Autodesk Inventor part; units mm, degrees
ref_plane "YZ Plane" through (0, 0, 0) normal (1, 0, 0) x (0, 1, 0)
ref_plane "XZ Plane" through (0, 0, 0) normal (0, 1, 0) x (-1, 0, 0)
ref_plane "XY Plane" through (0, 0, 0) normal (0, 0, 1) x (1, 0, 0)
sketch "Sketch1" plane through (0, 0, 0) normal (0, 1, 0) x (-1, 0, 0)
  point P0 (0, 0)
sketch "Sketch2" plane through (0, 0, 0) normal (0, 1, 0) x (-1, 0, 0)
  line L0 (38.1, 25.4) -> (-38.1, 25.4)
  line L1 (-38.1, 25.4) -> (-38.1, -25.4)
  line L2 (-38.1, -25.4) -> (38.1, -25.4)
  line L3 (38.1, -25.4) -> (38.1, 25.4)
  line L4 (34.798, 22.098) -> (-34.798, 22.098)
  line L5 (-34.798, 22.098) -> (-34.798, -22.098)
  line L6 (-34.798, -22.098) -> (34.798, -22.098)
  line L7 (34.798, -22.098) -> (34.798, 22.098)
  line L8 (0, -35.56) -> (0, 35.56)
  line L9 (-53.34, 0) -> (53.34, 0)
  point P0 (0, 0)
  dimension "d0" = 3.302
  dimension "d1" = 76.2
  dimension "d2" = 50.8
extrude "Extrusion1" add sketch "Sketch2" along normal mid plane 50.8 contours L3 L9 L7 L4 L8 L0 | L8 L4 L5 L9 L1 L0 | L3 L2 L8 L6 L7 L9 | L9 L5 L6 L8 L2 L1
sketch "Sketch3" plane through (-38.1, -25.4, 25.4) normal (0, 0, 1) x (1, 0, 0)
  circle A0 centre (25.4, 25.4) radius 14.2875
  line L0 (-15.24, 25.4) -> (91.44, 25.4)
  line L1 (38.1, 60.96) -> (38.1, -10.16)
  line L2 (0, 50.8) -> (0, 0)
  point P0 (38.1, 25.4)
  dimension "d5" = 28.575
  dimension "d6" = 25.4
extrude "Extrusion2" cut sketch "Sketch3" against normal up to surface (50.8 mm away)
properties part number "Hinge"
Could you check a few things on this model? Use its own coordinates, in mm. A direction names the side the tool comes from. Give positions to 0.01 mm unless a question says otherwise; leave off trailing zeros. Order: outer loops, then holes, each group sorted by start corner. A loop starts at its lowest first (then second) coordinate and runs counter-clockwise, first axis right, second up.
Q1. For faces 1 (the flat face through (8, 0, 25.4)), 2 (the flat face through (-34.798, 0, 0)), which set-ups out of +Z, -Z, +X, -X, +Y, -Y let a thin tool reach every point of the face, with its end or its side?
Q2. Suppose I cut it at A-A, the plane z = 4.5. Write out the boundary of the cut face in (x, y).
Q3. Suppose I cut it at B-B, the plane x = 8. Write out the boundary of the cut face in (y, z).
Q4. Suppose I cut it at C-C, the plane y = 0. Write out the boundary of the cut face in (x, z).
Q5. Suppose I cut it at D-D, the plane y = 20. Write out the boundary of the cut face in (x, z), and give its area (3 significant figures).
Q6. We'd pull the mould along Y, two halves only. Please class faces 3 (the cylindrical face through (0.93, 4.29, 23.77)), 4 (the cylindrical face through (0.93, 4.29, -23.73)), 5 (the flat face through (3, 25.4, -22.5)), 6 (the flat face through (38.1, 0, 0)): +Y half, -Y half, draft (parallel to the pull), parting line (faces both ways), or undercut.
Q7. If I drill on line 1 along Z through (x, y) = (27.5, 21); line 2 along X through (y, z) = (-11, -4.5); line 3 along X through (y, z) = (0, 23), over which ranges is the centre line in solid material (lowest first)?
Solution:
1. face 1: +Z, +X, -X, +Y, -Y
1. face 2: +Y, -Y
2. outline: (-38.1, -25.4) - (-34.8, -25.4) - (-34.8, 25.4) - (-38.1, 25.4) - close; (34.8, -25.4) - (38.1, -25.4) - (38.1, 25.4) - (34.8, 25.4) - close
3. outline: (-25.4, -25.4) - (25.4, -25.4) - (25.4, -22.1) - (-25.4, -22.1) - close; (-25.4, 22.1) - (25.4, 22.1) - (25.4, 25.4) - (-25.4, 25.4) - close
4. outline: (-38.1, -25.4) - (-26.99, -25.4) - (-26.99, -22.1) - (-34.8, -22.1) - (-34.8, 22.1) - (-26.99, 22.1) - (-26.99, 25.4) - (-38.1, 25.4) - close; (1.59, -25.4) - (38.1, -25.4) - (38.1, 25.4) - (1.59, 25.4) - (1.59, 22.1) - (34.8, 22.1) - (34.8, -22.1) - (1.59, -22.1) - close
5. outline: (-38.1, -25.4) - (38.1, -25.4) - (38.1, 25.4) - (-38.1, 25.4) - close; hole (-34.8, -22.1) - (34.8, -22.1) - (34.8, 22.1) - (-34.8, 22.1) - close
5. area: 795 mm2
6. face 3: undercut
6. face 4: undercut
6. face 5: +Y half
6. face 6: draft
7. line 1: z = -25.4 to -22.1, 22.1 to 25.4
7. line 2: x = -38.1 to -34.8, 34.8 to 38.1
7. line 3: x = -38.1 to -26.99, 1.59 to 38.1
